```python
from build123d import *

# Parameters (mm, degrees)
F1_DEPTH = 10
F2_R     = 5
F3_DEPTH = 18
F4_R     = 25.25
F4_R_2   = 5
F5_DEPTH = 10


with BuildPart() as f1:
    # F0 (on Front) → F1 (new body)
    with BuildSketch(Plane.XZ):
        Polygon((2.3851137612, 14.2932031622), (0, 7.5944172762), (-2.3851137612, 14.2932031622), (-2.4659032585, 7.1829308005), (-6.8968771988, 12.7443128177), (-4.6645876365, 5.9930623179), (-10.6612569758, 9.814378431), (-6.3577915656, 4.1537525412), (-13.270324133, 5.8209038555), (-7.3620301272, 1.8643192246), (-14.4413457601, 1.1966440267), (-7.5684784909, -0.6271420079), (-14.0474234935, -3.5572907503), (-6.954764773, -3.0506426728), (-12.1312449232, -7.9257378774), (-5.5873943777, -5.1435588684), (-8.9004577298, -11.4353083251), (-3.6145431043, -6.6790906501), (-4.7051678366, -13.7056856786), (-1.25, -7.4908393232), (0, -14.4908393232), (1.25, -7.4908393232), (4.7051678366, -13.7056856786), (3.6145431043, -6.6790906501), (8.9004577298, -11.4353083251), (5.5873943777, -5.1435588684), (12.1312449232, -7.9257378774), (6.954764773, -3.0506426728), (14.0474234935, -3.5572907503), (7.5684784909, -0.6271420079), (14.4413457601, 1.1966440267), (7.3620301272, 1.8643192246), (13.270324133, 5.8209038555), (6.3577915656, 4.1537525412), (10.6612569758, 9.814378431), (4.6645876365, 5.9930623179), (6.8968771988, 12.7443128177), (2.4659032585, 7.1829308005), align=None)
    extrude(amount=F1_DEPTH)

    # F2 (on face) → F3 (join)
    with BuildSketch(Plane.XZ.offset(10)):
        Circle(F2_R)
    extrude(amount=F3_DEPTH)

    # F4 (on face) → F5 (join)
    with BuildSketch(Plane.XZ.offset(28)):
        Circle(F4_R)
        Circle(F4_R_2, mode=Mode.SUBTRACT)
        Circle(F4_R_2)
    extrude(amount=F5_DEPTH)


solid = f1.part
```
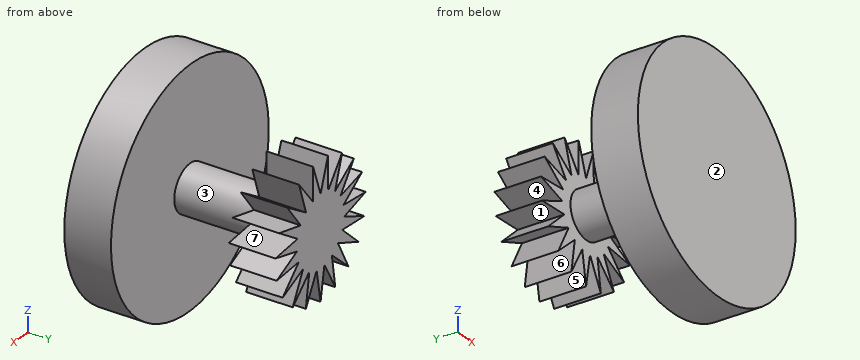
Could you check a few things on this model? Use its own coordinates, in mm. Face numbers are marked on the shaded views. A direction names the side the tool comes from. Give positions to 0.01 mm unless a question says otherwise; leave off trailing zeros. Loops run counter-clockwise (first coordinate to the right, second up) from the corner with the lowest first, then second, coordinate; pieces in that order, holes last. Notation, with made-up numbers: (41.5, -18.75) - (62.5, -18.75) arc R20 cw to (62.5, 0.25) - close; hole circle Ø3 at (-24, 73.25). An arc over 180 degrees is marked (long way). Use one line per item in the form item = value.
1. I want a section at A-A (y = -14). Please give me the cut outline in (x, z).
Response values:
outline = circle Ø10 at (0, 0)
2. I need wall thicknesses on probe 1 along X at (y, z) = (-6.5, -5.5); probe 2 along Y at (x, z) = (-7.5, 15); probe 3 along Z at (x, y) = (-3, -23.5). Which ranges of each line are inside material? Lowest first, please.
Response values:
probe_1 = -9.56 to -6.43, -5.78 to 5.78, 6.43 to 9.56
probe_2 = -38 to -28
probe_3 = -4 to 4
3. I want a section at C-C (x = 16.5). Please give me the cut outline in (y, z), and give its area (3 significant figures).
Response values:
outline = (-38, -19.11) - (-28, -19.11) - (-28, 19.11) - (-38, 19.11) - close
area = 382 mm²
4. I'm going to push flat-ended pins straight in: pin 1 Ø10 at (y, z) = (-13, 0.5) entering from -X; pin 2 Ø8 at (x, y) = (-4, -26.5) entering from +Z; pin 3 Ø1 at (x, z) = (8, 17) entering from +Y; pin 4 Ø12 at (y, z) = (-15, 18) entering from +X. Where does each tip first touch, or does it pass through?
Response values:
pin_1 = -14.44
pin_2 = 25.25
pin_3 = -28
pin_4 = through
5. Thinking about a two-plate mould opening in Z: for the marked faces 1, 2 and 3, which applies, released by +Z, released by -Z, zero draft, split by the parting line, or undercut?
Response values:
face_1 = undercut
face_2 = zero draft
face_3 = split by the parting line
6. On a 3-axis mill with a long thin cutter (end or side, diameter ignored), from which of +Z, -Z, +X, -X, +Y, -Y can I reach the whole of each face in a straight line? I mean the marked faces 4, 5, 6 and 7. Say none if no direction works.
Response values:
face_4 = -X, +Y
face_5 = -Z, +Y
face_6 = +Y
face_7 = +X, +Y
7. I want a section at B-B (x = -19.5). Please give me the cut outline in (y, z), and give its area (3 significant figures).
Response values:
outline = (-38, -16.04) - (-28, -16.04) - (-28, 16.04) - (-38, 16.04) - close
area = 321 mm²
